CAD build for the part. Positions are in the model's coordinates, mm. Face numbers are marked on the shaded views. A direction names the side the tool comes from. Round coordinates to 2 decimals unless told otherwise and drop trailing zeros. Order: outer loops, then holes, each group sorted by start corner. A loop starts at its lowest first (then second) coordinate and runs counter-clockwise, first axis right, second up. Notation, with made-up numbers: (25.25, 6.25) - (48.25, 6.25) arc R25 ccw to (48.25, 18.25) - close; hole circle Ø8 at (24.25, 2.5). An arc over 180 degrees is marked (long way). Write item = value, one per line.
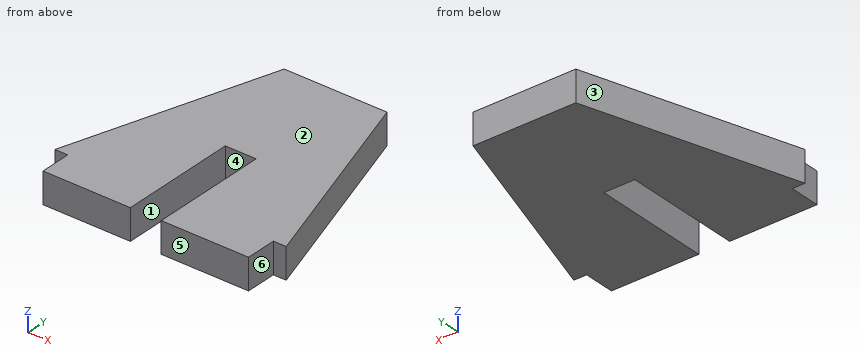
from build123d import *

# Parameters (mm, degrees)
BOSS_EXTRUDE1_DEPTH = 3
SKETCH2_W           = 6
SKETCH2_H           = 23
CUT_EXTRUDE1_DEPTH  = 7


with BuildPart() as part:
    # Sketch1 → Boss-Extrude1 (new body, symmetric)
    with BuildSketch(Plane.XY):
        Polygon((-20, 0), (20, 0), (20, 6), (22.5, 6), (10, 46), (-10, 46), (-22.5, 6), (-20, 6), align=None)
    extrude(amount=BOSS_EXTRUDE1_DEPTH, both=True)

    # Sketch2 → Cut-Extrude1 (cut, through all)
    with BuildSketch(Plane.XY.offset(3)):
        with Locations((0, 11.5)):
            Rectangle(SKETCH2_W, SKETCH2_H)
    extrude(amount=-CUT_EXTRUDE1_DEPTH, mode=Mode.SUBTRACT)


solid = part.part
(1) Pull direction X, two halves, no side cores. Call the marked faces 3, 4, 5 and 6: released by +X, released by -X, zero draft, split by the parting line, or undercut.
Solved:
face_3 = released by -X
face_4 = undercut
face_5 = zero draft
face_6 = released by +X
(2) Band-saw the part on C-C on x = -17. List the corners of the cut face in (y, z), plus the area to 3 significant figures.
Solved:
outline = (0, -3) - (23.6, -3) - (23.6, 3) - (0, 3) - close
area = 142 mm²
(3) Band-saw the part on B-B on y = 20.5. List the corners of the cut face in (x, z), plus the area to 3 significant figures.
Solved:
outline = (-17.97, -3) - (-3, -3) - (-3, 3) - (-17.97, 3) - close; (3, -3) - (17.97, -3) - (17.97, 3) - (3, 3) - close
area = 180 mm²
(4) Probe line 1 along X through (y, z) = (4.5, -0.6); line 2 along Y through (x, z) = (-1, 0.4); line 3 along X through (y, z) = (12.5, 2.4). List the from-to ranges inside material, lowest first.
Solved:
line_1 = -20 to -3, 3 to 20
line_2 = 23 to 46
line_3 = -20.47 to -3, 3 to 20.47
(5) Band-saw the part on A-A on z = 0.95. List the corners of the cut face in (x, y).
Solved:
outline = (-22.5, 6) - (-20, 6) - (-20, 0) - (-3, 0) - (-3, 23) - (3, 23) - (3, 0) - (20, 0) - (20, 6) - (22.5, 6) - (10, 46) - (-10, 46) - close
(6) Tool access for the marked faces 1 and 2: list every direction of +Z, -Z, +X, -X, +Y, -Y with a clear straight run to the whole face (end or side of a thin tool).
Solved:
face_1 = +Z, -Z, -Y
face_2 = +Z, +X, -X, +Y, -Y
(7) Band-saw the part on D-D on y = 41. List the corners of the cut face in (x, z).
Solved:
outline = (-11.56, -3) - (11.56, -3) - (11.56, 3) - (-11.56, 3) - close
(8) Drop flat-ended pins along their axis: pin 1 (1.2 mm diameter, centred on x = -22, z = -1, fed in from -Y); pin 2 (1.8 mm diameter, centred on x = -0.5, z = -1, fed in from -Y); pin 3 (1.8 mm diameter, centred on y = 4.5, z = -1, fed in from -X); pin 4 (1 mm diameter, centred on x = -9, z = -2, fed in from -Y). Give the stop position or say it passes through.
Solved:
pin_1 = 6
pin_2 = 23
pin_3 = -20
pin_4 = 0
